Work out the finished part from the listing and answer in its coordinate system (mm). A direction names the side the tool comes from. Coordinates: 2 decimals unless noted, no trailing zeros. Write each loop counter-clockwise with the first axis right and the second up, starting at its lowest first coordinate (ties: lowest second). Pieces come first, ordered by that corner, then holes. Notation, with made-up numbers: (48, 1) - (104, 1) arc R12 cw to (104, 6) - close; hole circle Ø1 at (-36, 88). An arc over 180 degrees is marked (long way). Use one line per item in the form item = value. Start each with the question number.
Item 1: A cutting plane is placed at B-B (x = -16.5). Write down the section's boundary in (y, z).
Item 2: Given pin 1 (12 mm diameter, centred on y = 15, z = 41, fed in from +X); pin 2 (6 mm diameter, centred on y = 39.5, z = 35.5, fed in from -X); pin 3 (2 mm diameter, centred on x = -13, y = 9, fed in from +Z); pin 4 (0.9 mm diameter, centred on x = -12, z = 29.5, fed in from -Y), each flat-ended and moving along its own axis, determine where each tip first touches the part or whether it passes through.
Item 3: A cutting plane is placed at A-A (x = -13). Write down the section's boundary in (y, z), then the cut area to 3 significant figures.
Item 4: A cutting plane is placed at C-C (z = 18). Write down the section's boundary in (x, y), then the cut area to 3 significant figures.
Item 5: A cutting plane is placed at D-D (y = 14.5). Write down the section's boundary in (x, z), then the cut area to 3 significant figures.
Item 6: For faces 1 (the flat face through (-12, 26.589, 30)), 2 (the flat face through (-12, 46.589, 26)), determine the directions among +Z, -Z, +X, -X, +Y, -Y from which every point of the face is accessible in a straight line to the end or side of a thin tool.
Item 7: Consider probe 1 along Y at (x, z) = (-14, 5); probe 2 along Y at (x, z) = (-14.75, 5); probe 3 along Y at (x, z) = (-11.65, 46). Determine where each line is inside the solid, lowest interval first.
Autodesk Inventor part; units mm, degrees
ref_plane "YZ Plane" through (0, 0, 0) normal (1, 0, 0) x (0, 1, 0)
ref_plane "XZ Plane" through (0, 0, 0) normal (0, 1, 0) x (-1, 0, 0)
ref_plane "XY Plane" through (0, 0, 0) normal (0, 0, 1) x (1, 0, 0)
sketch "Sketch1" plane through (0, 0, 0) normal (0, 0, 1) x (1, 0, 0)
  line L0 (-17.8598, 36.5888) -> (-10.8598, 36.5888)
  line L1 (-10.8598, 36.5888) -> (-10.8598, -13.4112)
  line L2 (-10.8598, -13.4112) -> (-17.8598, -13.4112)
  line L3 (-17.8598, -13.4112) -> (-17.8598, 36.5888)
  point P0 (0, 0)
  dimension "d0" = 7
  dimension "d1" = 50
extrude "Extrusion1" add sketch "Sketch1" along normal blind 10
sketch "Sketch2" plane through (-17.8598, -13.4112, 0) normal (-1, 0, 0) x (0, 0, 1)
  line L0 (0, 0) -> (10, 0)
  line L1 (0, 50) -> (0, 0)
  point P0 (0, 13.4112)
  point P1 (5, 10)
  point P2 (5, 40)
  dimension "d4" = 10
  dimension "d5" = 5
  dimension "d6" = 5
  dimension "d7" = 30
hole "Hole1" at (-17.8598, -3.4112, 5) at (-17.8598, 26.5888, 5) direction (1, 0, 0) diameter 3 depth 7 tip angle 118
chamfer "Chamfer1" distance 5 angle 45 1 edges at (-10.8598, -13.4112, 5)
sketch "Sketch3" plane through (-17.8598, -13.4112, 0) normal (-1, 0, 0) x (0, 0, 1)
  line L0 (0, 50) -> (51, 50)
  line L1 (51, 50) -> (51, 60)
  line L2 (51, 60) -> (0, 60)
  line L3 (0, 60) -> (0, 50)
  line L4 (10, 50) -> (10, 0)
  line L5 (10, 40) -> (51, 40)
  line L6 (51, 40) -> (51, 50)
  line L7 (51, 50) -> (10, 50)
  line L8 (10, 50) -> (10, 40)
  point P0 (0, 13.4112)
  dimension "d18" = 51
  dimension "d19" = 10
  dimension "d20" = 10
extrude "Extrusion2" add sketch "Sketch3" against normal blind 7
sketch "Sketch4" plane through (-17.8598, -13.4112, 0) normal (-1, 0, 0) x (0, 0, 1)
  line L0 (0, 60) -> (51, 60)
  line L1 (51, 40) -> (10, 40)
  line L2 (10, 40) -> (10, 60)
  line L3 (10, 60) -> (51, 60)
  line L4 (51, 60) -> (51, 40)
  line L5 (10, 40) -> (10, 0)
  line L6 (0, 60) -> (0, 5)
  line L7 (10, 60) -> (0, 60)
  line L8 (0, 60) -> (0, 45)
  line L9 (0, 45) -> (10, 45)
  line L10 (10, 45) -> (10, 60)
  point P0 (0, 13.4112)
  dimension "d23" = 15
extrude "Extrusion3" cut sketch "Sketch4" against normal blind 4
sketch "Sketch5" plane through (-13.8598, -13.4112, 0) normal (-1, 0, 0) x (0, 0, 1)
  line L0 (51, 60) -> (51, 40)
  line L1 (0, 45) -> (0, 60)
  line L2 (0, 60) -> (51, 60)
  point P0 (0, 13.4112)
  point P1 (5, 55)
  point P2 (46, 55)
  dimension "d26" = 5
  dimension "d27" = 5
  dimension "d28" = 5
  dimension "d29" = 5
hole "Hole2" at (-13.8598, 41.5888, 5) at (-13.8598, 41.5888, 46) direction (1, 0, 0) diameter 3 depth 7 tip angle 118 countersink diameter 6 countersink angle 90
chamfer "Chamfer2" distance 5 angle 45 2 edges at (-12.3598, 46.5888, 51) (-12.3598, 46.5888, 0)
chamfer "Chamfer3" distance 4 angle 45 1 edges at (-13.8598, 31.5888, 5)
sketch "Sketch6" plane through (-13.8598, -13.4112, 0) normal (-1, 0, 0) x (0, 0, 1)
  circle A0 centre (46, 55) radius 1.5
  circle A1 centre (5, 55) radius 1.5
  point P0 (0, 13.4112)
  dimension "d43" = 41
sketch "Sketch7" plane through (-13.8598, -13.4112, 0) normal (-1, 0, 0) x (0, 0, 1)
  line L0 (0, 49) -> (0, 55)
  circle A0 centre (5, 55) radius 1.5
  point P0 (0, 13.4112)
  dimension "d44" = 5
properties part number "Z-stepper connector"
Answer:
q1.outline = (-13.41, 0) - (32.95, 0) - (32.95, 10) - (-13.41, 10) - close; hole circle Ø3 at (-3.41, 5); hole circle Ø3 at (26.59, 5)
q2.pin_1 = through
q2.pin_2 = -13.86
q2.pin_3 = 10
q2.pin_4 = 26.59
q3.outline = (-10.55, 0) - (41.59, 0) - (46.59, 5) - (46.59, 46) - (41.59, 51) - (26.59, 51) - (26.59, 10) - (-10.55, 10) - close; hole circle Ø3 at (-3.41, 5); hole circle Ø3 at (26.59, 5); hole circle Ø4.28 at (41.59, 5); hole circle Ø4.28 at (41.59, 46)
q3.area = 1,320 mm²
q4.outline = (-13.86, 26.59) - (-10.86, 26.59) - (-10.86, 46.59) - (-13.86, 46.59) - close
q4.area = 60.0 mm²
q5.outline = (-17.86, 0) - (-10.86, 0) - (-10.86, 10) - (-17.86, 10) - close
q5.area = 70.0 mm²
q6.face_1 = +Z, +X, -X, -Y
q6.face_2 = +Z, -Z, +X, -X, +Y
q7.probe_1 = -11.55 to -4.91, -1.91 to 25.09, 28.09 to 35.45
q7.probe_2 = -12.3 to -4.91, -1.91 to 25.09, 28.09 to 34.7
q7.probe_3 = 26.59 to 40.09, 43.09 to 46.59
